Could you check a few things on this model? Use its own coordinates, in mm. A direction names the side the tool comes from. Give positions to 0.01 mm unless a question says otherwise; leave off trailing zeros. Loops run counter-clockwise (first coordinate to the right, second up) from the corner with the lowest first, then second, coordinate; pieces in that order, holes last. Notation, with made-up numbers: (0.25, 65) - (8.25, 65) arc R22 ccw to (8.25, 86) - close; hole circle Ø10 at (34.25, -33.5). An arc over 180 degrees is marked (long way). Write each question's results on one line, items separated by ' | '. Start each with the question number.
1) I want a section at A-A, the plane z = -23.5. Write out the boundary of the cut face in (x, y) (3 decimals), and give its area (3 significant figures).
2) If we mould it in two halves opening along Z, with no side actions, what happens to faces 1 (the face through (0, -34.925, 9)), 2 (the face through (6, -22.225, 0)), 3 (the face through (-0.12, 31.06, -5.34)), 4 (the face through (-1, 1, -38.1))? For each: +Z half, -Z half, draft (parallel to the pull), parting line (faces both ways), or undercut.
3) If I drill on probe 1 along X at (y, z) = (-10, 33.5) (3 decimals); probe 2 along Z at (x, y) = (27.5, -26.5) (3 decimals), over which ranges is the centre line in solid material (lowest first)? Write a range as [from, to].
4) I'm going to push flat-ended pins straight in: pin 1 (1 mm diameter, centred on x = -4.5, y = 24, fed in from +Z); pin 2 (3 mm diameter, centred on x = -7, y = -13, fed in from +Z) (3 decimals). Where does each tip first touch, or does it pass through?
5) On a 3-axis mill with a long thin cutter (end or side, diameter ignored), from which of +Z, -Z, +X, -X, +Y, -Y can I reach the whole of each face in a straight line? I mean faces 5 (the face through (-1, -38.1, -1)), 6 (the face through (0, 25, -1.588)), 7 (the face through (34.925, 0, 1)). Say none if no direction works.
6) I want a section at D-D, the plane z = -3. Write out the boundary of the cut face in (x, y) (1 decimal).
7) I want a section at B-B, the plane x = -24.5. Write out the boundary of the cut face in (y, z) (3 decimals).
from build123d import *

# Parameters (mm, degrees)
BOSS_EXTRUDE1_DEPTH      = 38.1
BOSS_EXTRUDE1_DEPTH_BACK = 38.1
SKETCH1_W                = 76.2
SKETCH1_H                = 76.2
SHELL1_T                 = -3.175
SKETCH2_W                = 16.51
SKETCH2_H                = 3.175
BOSS_EXTRUDE2_DEPTH      = 12.7
SKETCH3_R                = 1.27
SKETCH3_W                = 6.35
SKETCH3_H                = 2.54
CUT_EXTRUDE1_DEPTH       = 12.7
FILLET1_R                = 1.27
FILLET1_OF_MIRROR2_R     = 1.27
CHAMFER1_SIZE            = 7.62


with BuildPart() as part:
    # Sketch1 → Boss-Extrude1 (new, two sides: drawn at the far end of the back side and taken through both)
    with BuildSketch(Plane.XY.offset(-BOSS_EXTRUDE1_DEPTH_BACK)):
        Rectangle(SKETCH1_W, SKETCH1_H)
    extrude(amount=BOSS_EXTRUDE1_DEPTH + BOSS_EXTRUDE1_DEPTH_BACK)

    # Shell1
    shell1_openings = [part.faces().sort_by_distance(p)[0] for p in [
        (0, 0, 38.1),
    ]]
    offset(amount=SHELL1_T, openings=shell1_openings, kind=Kind.INTERSECTION)

    # Sketch2 → Boss-Extrude2 (add)
    with BuildSketch(Plane.XZ.offset(-34.925)):
        Rectangle(SKETCH2_W, SKETCH2_H)
    boss_extrude2 = extrude(amount=BOSS_EXTRUDE2_DEPTH)

    # Sketch3 → Cut-Extrude1 (cut, symmetric)
    with BuildSketch(Plane.XY.offset(1.5875)):
        with Locations(Location((-5.715, 24.765, 0), (0, 0, 180))):
            Circle(SKETCH3_R)
        with Locations(Location((5.715, 24.765, 0), (0, 0, 180))):
            Circle(SKETCH3_R)
        with Locations((0, 23.495)):
            Rectangle(SKETCH3_W, SKETCH3_H)
    cut_extrude1 = extrude(amount=CUT_EXTRUDE1_DEPTH, both=True, mode=Mode.SUBTRACT)

    # Fillet1
    fillet1_edges = [part.edges().sort_by_distance(p)[0] for p in [
        (-3.175, 24.765, 0),
        (8.255, 22.225, 0),
        (3.175, 22.225, 0),
        (-3.175, 22.225, 0),
        (-8.255, 22.225, 0),
        (3.175, 24.765, 0),
    ]]
    fillet(fillet1_edges, radius=FILLET1_R - 0.0001)  # a hair under: the kernel refuses the full size

    # Mirror2: Boss-Extrude2, Cut-Extrude1 across plane
    add(boss_extrude2.mirror(Plane.ZX))
    add(cut_extrude1.mirror(Plane.ZX), mode=Mode.SUBTRACT)

    # Fillet1 of Mirror2
    fillet1_of_mirror2_edges = [part.edges().sort_by_distance(p)[0] for p in [
        (-3.175, -24.765, 0),
        (8.255, -22.225, 0),
        (3.175, -22.225, 0),
        (-3.175, -22.225, 0),
        (-8.255, -22.225, 0),
        (3.175, -24.765, 0),
    ]]
    fillet(fillet1_of_mirror2_edges, radius=FILLET1_OF_MIRROR2_R - 0.0001)  # a hair under: the kernel refuses the full size

    # Chamfer1
    chamfer1_edges = [part.edges().sort_by_distance(p)[0] for p in [
        (0, -34.925, -1.5875),
        (0, 34.925, -1.5875),
    ]]
    chamfer(chamfer1_edges, length=CHAMFER1_SIZE)


solid = part.part
Answers:
1) outline: (-38.1, -38.1) - (38.1, -38.1) - (38.1, 38.1) - (-38.1, 38.1) - close; hole (-34.925, -34.925) - (34.925, -34.925) - (34.925, 34.925) - (-34.925, 34.925) - close | area: 927 mm2
2) face 1: undercut | face 2: draft | face 3: undercut | face 4: -Z half
3) probe 1: x = [-38.1, -34.925], [34.925, 38.1] | probe 2: z = [-38.1, -34.925]
4) pin 1: stops at z = 1.59 | pin 2: stops at z = -34.925
5) face 5: +Z, -Z, +X, -X, -Y | face 6: none | face 7: +Z
6) outline: (-38.1, -38.1) - (38.1, -38.1) - (38.1, 38.1) - (-38.1, 38.1) - close; hole (-34.9, -34.9) - (-8.3, -34.9) - (-8.3, -28.7) - (8.3, -28.7) - (8.3, -34.9) - (34.9, -34.9) - (34.9, 34.9) - (8.3, 34.9) - (8.3, 28.7) - (-8.3, 28.7) - (-8.3, 34.9) - (-34.9, 34.9) - close
7) outline: (-38.1, -38.1) - (38.1, -38.1) - (38.1, 38.1) - (34.925, 38.1) - (34.925, -34.925) - (-34.925, -34.925) - (-34.925, 38.1) - (-38.1, 38.1) - close
